Source: CAD feature listing. Evaluate the final solid. Frame: model axes, mm. A direction names the side the tool comes from. Give positions to 0.01 mm unless a question says otherwise; leave off trailing zeros. Loops run counter-clockwise (first coordinate to the right, second up) from the corner with the lowest first, then second, coordinate; pieces in that order, holes last. Notation, with made-up numbers: (71.5, 46) -> (130.5, 46) arc R26 ccw to (130.5, 70) -> close; hole circle Ø1 at (70.25, 34.25). An arc over 180 degrees is marked (long way). Put each result on its own line as item: value.
```python
from build123d import *

# Parameters (mm, degrees)
SKETCH1_R                 = 12.5
BOSS_EXTRUDE1_DEPTH       = 27.94
SKETCH2_R                 = 6
BOSS_EXTRUDE2_DEPTH       = 2
SKETCH3_R                 = 2
BOSS_EXTRUDE3_DEPTH       = 10
M3X0_5_TAPPED_HOLE1_D     = 2.5
M3X0_5_TAPPED_HOLE1_DEPTH = 3.999992
M3X0_5_TAPPED_HOLE1_TIP   = 0.751075774
FILLET1_R                 = 1.27


with BuildPart() as part:
    # Sketch1 → Boss-Extrude1 (new body)
    with BuildSketch(Plane.XY):
        Circle(SKETCH1_R)
    extrude(amount=BOSS_EXTRUDE1_DEPTH)

    # Sketch2 → Boss-Extrude2 (add)
    with BuildSketch(Plane.XY.offset(27.94)):
        Circle(SKETCH2_R)
    extrude(amount=BOSS_EXTRUDE2_DEPTH)

    # Sketch3 → Boss-Extrude3 (add)
    with BuildSketch(Plane.XY.offset(29.94)):
        Circle(SKETCH3_R)
    extrude(amount=BOSS_EXTRUDE3_DEPTH)

    # M3x0.5 Tapped Hole1
    with Locations(Plane.XY.offset(27.94)):
        with Locations((-9, 0), (9, 0)):
            Hole(M3X0_5_TAPPED_HOLE1_D / 2, depth=M3X0_5_TAPPED_HOLE1_DEPTH)
            with Locations((0, 0, -(M3X0_5_TAPPED_HOLE1_DEPTH + M3X0_5_TAPPED_HOLE1_TIP / 2))):  # 118° drill point
                Cone(0, M3X0_5_TAPPED_HOLE1_D / 2, M3X0_5_TAPPED_HOLE1_TIP, mode=Mode.SUBTRACT)

    # Fillet1
    fillet1_edges = [part.edges().sort_by_distance(p)[0] for p in [
        (-12.5, 0, 0),
    ]]
    fillet(fillet1_edges, radius=FILLET1_R)


solid = part.part
```
(1) Reachability of faces 1 (the cylindrical face through (0, -2, 35)), 2 (the flat face through (0, 0, 39.94)) from +Z, -Z, +X, -X, +Y, -Y: full face, straight path, thin tool, end or side. Return the list, or none.
Calculated:
face 1: +Z
face 2: +Z, +X, -X, +Y, -Y
(2) First-contact query: P1, Ø1, axis at y = -2, z = 30.5, coming from the -X side; P2, Ø10, axis at x = -4, z = 35.5, coming from the -Y side; P3, Ø6, axis at y = 4.5, z = 28, coming from the -X side. Flat tips, straight axial feed; report the tip coordinate or a pass-through.
Calculated:
P1: stops at x = -1.32
P2: stops at y = -2
P3: stops at x = -12.41
(3) Section A-A on x = 0. Return loops of the section in (y, z).
Calculated:
outline: (-12.5, 1.27) arc R1.27 ccw to (-11.23, 0) -> (11.23, 0) arc R1.27 ccw to (12.5, 1.27) -> (12.5, 27.94) -> (6, 27.94) -> (6, 29.94) -> (2, 29.94) -> (2, 39.94) -> (-2, 39.94) -> (-2, 29.94) -> (-6, 29.94) -> (-6, 27.94) -> (-12.5, 27.94) -> close
(4) Section B-B on z = 17. Return loops of the section in (x, y), then the cut area to 3 significant figures.
Calculated:
outline: circle Ø25 at (0, 0)
area: 491 mm²
(5) Line query: probe 1 along Z at (x, y) = (8, 2.75); probe 2 along Z at (x, y) = (-4, -3.5); probe 3 along Y at (x, z) = (-9, 24.9). Output: solid intervals per line, ascending. Write a range as from..to.
Calculated:
probe 1: z = 0..27.94
probe 2: z = 0..29.94
probe 3: y = -8.67..-1.25, 1.25..8.67
(6) Draft query along Y for faces 3 (the flat face through (-3, -5.4, 27.94)), 4 (the cylindrical face through (-7.75, 0.05, 25.91)), 5 (the cylindrical face through (11.923, 3.755, 14.418)). Return one class per face: released by +Y, released by -Y, zero draft, split by the parting line, or undercut.
Calculated:
face 3: zero draft
face 4: undercut
face 5: split by the parting line
